CAD build for the part. Positions are in the model's coordinates, mm. A direction names the side the tool comes from. Coordinates: 2 decimals unless noted, no trailing zeros. Order: outer loops, then holes, each group sorted by start corner. A loop starts at its lowest first (then second) coordinate and runs counter-clockwise, first axis right, second up. Notation, with made-up numbers: M 35.25,-26 L 81.25,-26 A20 cw 81.25,0 Z; hole C -4.5,-25 d8. An arc over 180 degrees is marked long. Write item = value, one per line. Start each with the question number.
```python
from build123d import *

# Parameters (mm, degrees)
PAD_DEPTH    = 3
SKETCH001_W  = 15.3
SKETCH001_H  = 15.3
SKETCH001_R  = 5.7
PAD001_DEPTH = 6
SKETCH002_R  = 5
PAD002_DEPTH = 15
SKETCH003_R  = 1.58
POCKET_DEPTH = 8
FILLET_R     = 2


with BuildPart() as part:
    # Sketch → Pad (new body)
    with BuildSketch(Plane.XY):
        Polygon((-9.25, 6.75), (-6.75, 9.25), (6.75, 9.25), (9.25, 6.75), (9.25, -6.75), (6.75, -9.25), (-6.75, -9.25), (-9.25, -6.75), align=None)
    extrude(amount=PAD_DEPTH)

    # Sketch001 → Pad001 (new body)
    with BuildSketch(Plane.XY.offset(3)):
        Rectangle(SKETCH001_W, SKETCH001_H)
        Circle(SKETCH001_R, mode=Mode.SUBTRACT)
    extrude(amount=PAD001_DEPTH)

    # Sketch002 → Pad002 (new body)
    with BuildSketch(Plane(origin=(0, 0, 0), x_dir=(1, 0, 0), z_dir=(0, 0, -1))):
        Circle(SKETCH002_R)
    extrude(amount=PAD002_DEPTH)

    # Sketch003 → Pocket (cut)
    with BuildSketch(Plane(origin=(0, 0, -15), x_dir=(1, 0, 0), z_dir=(0, 0, -1))):
        Circle(SKETCH003_R)
    extrude(amount=-POCKET_DEPTH, mode=Mode.SUBTRACT)

    # Fillet
    fillet_edges = [part.edges().sort_by_distance(p)[0] for p in [
        (-7.65, -7.65, 6),
        (7.65, -7.65, 6),
        (-7.65, 7.65, 6),
        (7.65, 7.65, 6),
    ]]
    fillet(fillet_edges, radius=FILLET_R)


solid = part.part
```
1. Flat gauge pins, fed straight in: pin 1 (6 mm diameter, centred on x = -2.5, z = 4, fed in from +Y); pin 2 (3 mm diameter, centred on x = 0, y = 0, fed in from +Z); pin 3 (1.8 mm diameter, centred on y = -2, z = 4.5, fed in from -X); pin 4 (1 mm diameter, centred on x = 2.5, z = -1.5, fed in from +Y). Where does each tip first touch, or does it go through?
2. Probe L1, parallel to Y at x = 0, z = -12.75; L2, parallel to Y at x = 0, z = 4.9; L3, parallel to Z at x = 6, y = -6. List the from-to ranges inside material, lowest first.
3. Slice it at A-A (z = 7.5). Write the cut outline in (x, y), plus the area to 3 significant figures.
4. Mould opens along Y. For faces 6 (the flat face through (0, -8, 3)), 7 (the flat face through (0, 0, -7)), 8 (the flat face through (-8, 8, 1)) say: released by +Y, released by -Y, zero draft, split by the parting line, or undercut.
5. Slice it at D-D (z = -3). Write the cut outline in (x, y), plus the area to 3 significant figures.
6. Slice it at B-B (y = 0). Write the cut outline in (x, z), plus the area to 3 significant figures.
7. 3-axis set-ups, long thin cutter, end or side, ignore diameter. For faces 1 (the cylindrical face through (-7.08, 7.05, 6.04)), 2 (the flat face through (0, 0, 3)), 3 (the cylindrical face through (-1.08, 4.88, -7.4)), 4 (the flat face through (0, 7.65, 6)), 5 (the flat face through (-7.65, 0, 6)): which of +Z, -Z, +X, -X, +Y, -Y reach the whole face in a straight line?
Calculated:
q1.pin_1 = 9.25
q1.pin_2 = 3
q1.pin_3 = -7.65
q1.pin_4 = 4.58
q2.L1 = -5 to -1.58, 1.58 to 5
q2.L2 = -7.65 to -5.7, 5.7 to 7.65
q2.L3 = 0 to 9
q3.outline = M -7.65,-5.65 A2 ccw -5.65,-7.65 L 5.65,-7.65 A2 ccw 7.65,-5.65 L 7.65,5.65 A2 ccw 5.65,7.65 L -5.65,7.65 A2 ccw -7.65,5.65 Z; hole C 0,0 d11.4
q3.area = 129 mm²
q4.face_6 = zero draft
q4.face_7 = undercut
q4.face_8 = released by +Y
q5.outline = C 0,0 d10
q5.area = 78.5 mm²
q6.outline = M -9.25,0 L -5,0 L -5,-15 L -1.58,-15 L -1.58,-7 L 1.58,-7 L 1.58,-15 L 5,-15 L 5,0 L 9.25,0 L 9.25,3 L 7.65,3 L 7.65,9 L 5.7,9 L 5.7,3 L -5.7,3 L -5.7,9 L -7.65,9 L -7.65,3 L -9.25,3 Z
q6.area = 204 mm²
q7.face_1 = +Z, -X, +Y
q7.face_2 = +Z
q7.face_3 = -Z
q7.face_4 = +Z, +X, -X, +Y
q7.face_5 = +Z, -X, +Y, -Y
